Check sheet for the drawn part. Datum: minimum x, y, z corner. Units: mm. A direction names the side the tool comes from. Give positions to 0.01 mm unless a question says otherwise; leave off trailing zeros. Write each loop counter-clockwise with the first axis right and the second up, starting at its lowest first coordinate (ties: lowest second). Pieces come first, ordered by that corner, then holes.
(1) Depth check by flat-ended pin: P1, Ø10, axis at y = 9.5, z = 22, coming from the +X side; P2, Ø3, axis at x = 16, y = 10.5, coming from the +Z side; P3, Ø1.5, axis at x = 12.5, y = 5.5, coming from the -Z side; P4, Ø1, axis at x = 20, z = 7.5, coming from the -Y side. Enter the tip coordinate at first touch or a pass-through.
(2) Tool access check on the marked faces 4 and 5. Record the directions out of +Z, -Z, +X, -X, +Y, -Y that give a thin tool (end or side, any length) a straight path to the whole face; none if there is none.
(3) Cross-section at B-B (x = 12.5). Record the boundary of the cut face in (y, z), and give its area (3 significant figures).
(4) Mould release check, pull along Z, two halves, no side actions. Record for the marked faces 1, 2 and 3: +Z half, -Z half, draft (parallel to the pull), parting line (faces both ways), or undercut.
(5) Cross-section at D-D (z = 5.75). Record the boundary of the cut face in (x, y).
(6) Thickness scan on line 1 along Y through (x, z) = (14.25, 5); line 2 along X through (y, z) = (6, 13.75); line 3 along Z through (x, y) = (18, 2). Record the ranges inside material, lowest first.
(7) Cross-section at C-C (y = 13.5). Record the boundary of the cut face in (x, z), and give its area (3 significant figures).
(8) Cross-section at A-A (z = 12.5). Record the boundary of the cut face in (x, y).
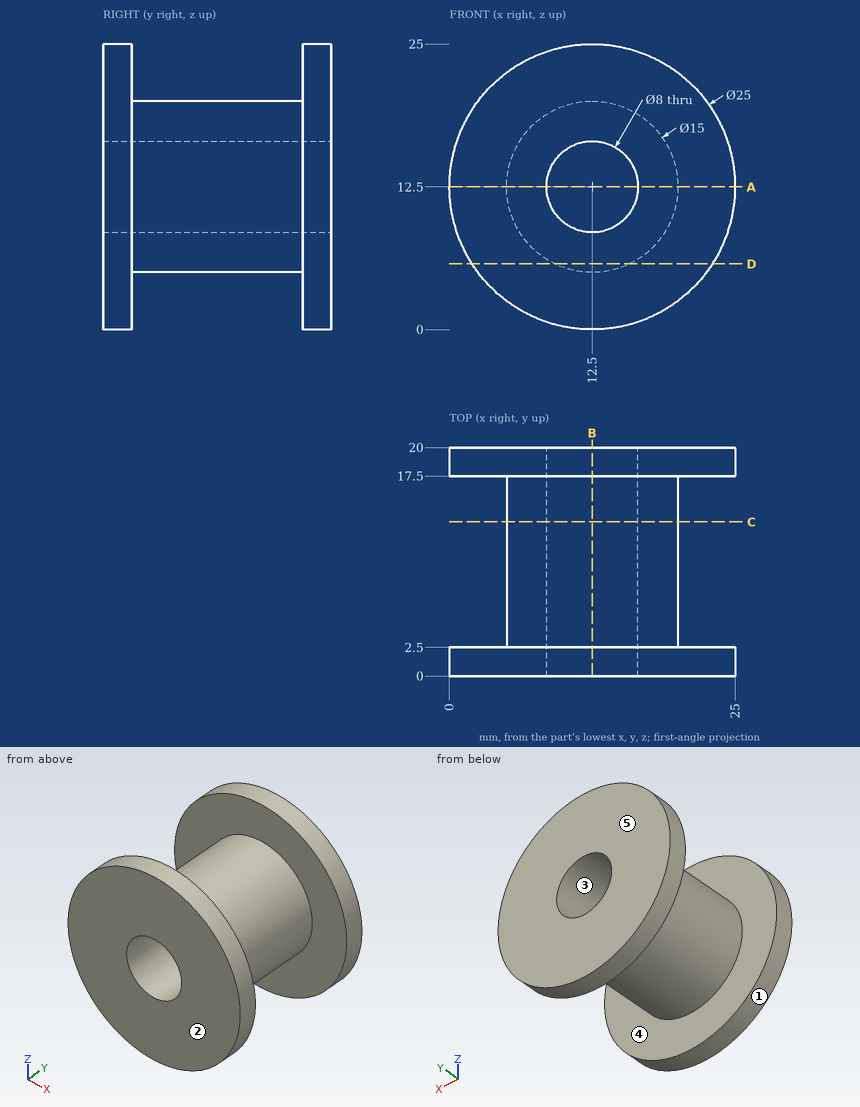
Reply:
1. P1: stops at x = 18.5
1. P2: stops at z = 19.73
1. P3: stops at z = 5
1. P4: stops at y = 0
2. face 4: none
2. face 5: +Z, -Z, +X, -X, +Y
3. outline: (0, 0) - (2.5, 0) - (2.5, 5) - (17.5, 5) - (17.5, 0) - (20, 0) - (20, 8.5) - (0, 8.5) - close; (0, 16.5) - (20, 16.5) - (20, 25) - (17.5, 25) - (17.5, 20) - (2.5, 20) - (2.5, 25) - (0, 25) - close
3. area: 190 mm2
4. face 1: parting line
4. face 2: draft
4. face 3: undercut
5. outline: (1.98, 0) - (23.02, 0) - (23.02, 2.5) - (15.77, 2.5) - (15.77, 17.5) - (23.02, 17.5) - (23.02, 20) - (1.98, 20) - (1.98, 17.5) - (9.23, 17.5) - (9.23, 2.5) - (1.98, 2.5) - close
6. line 1: y = 0 to 2.5, 17.5 to 20
6. line 2: x = 5.1 to 8.7, 16.3 to 19.9
6. line 3: z = 1.28 to 23.72
7. outline: circle Ø15 at (12.5, 12.5); hole circle Ø8 at (12.5, 12.5)
7. area: 126 mm2
8. outline: (0, 0) - (8.5, 0) - (8.5, 20) - (0, 20) - (0, 17.5) - (5, 17.5) - (5, 2.5) - (0, 2.5) - close; (16.5, 0) - (25, 0) - (25, 2.5) - (20, 2.5) - (20, 17.5) - (25, 17.5) - (25, 20) - (16.5, 20) - close
